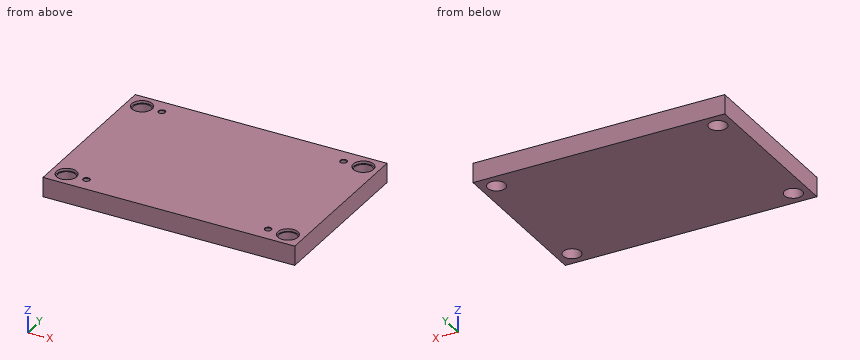
from build123d import *

# Parameters (mm, degrees)
SZKIC1_W                    = 596
SZKIC1_H                    = 396
DODANIE_WYCI_GNI_CIE1_DEPTH = 46
SZKIC2_R                    = 21
WYTNIJ_WYCI_GNI_CIE1_DEPTH  = 46
SZKIC3_R                    = 21
WYTNIJ_WYCI_GNI_CIE2_DEPTH  = 46
SZKIC4_R                    = 21
WYTNIJ_WYCI_GNI_CIE3_DEPTH  = 46
SZKIC5_R                    = 21
WYTNIJ_WYCI_GNI_CIE4_DEPTH  = 46
SZKIC6_R                    = 24
WYTNIJ_WYCI_GNI_CIE5_DEPTH  = 6.3
SZKIC7_R                    = 24
WYTNIJ_WYCI_GNI_CIE6_DEPTH  = 6.3
SZKIC8_R                    = 24
WYTNIJ_WYCI_GNI_CIE7_DEPTH  = 6.3
SZKIC9_R                    = 24
WYTNIJ_WYCI_GNI_CIE8_DEPTH  = 6.3


with BuildPart() as part:
    # Szkic1 → Dodanie-wyci_gni_cie1 (new body)
    with BuildSketch(Plane.XY):
        Rectangle(SZKIC1_W, SZKIC1_H)
    extrude(amount=DODANIE_WYCI_GNI_CIE1_DEPTH)

    # Szkic2 → Wytnij-wyci_gni_cie1 (cut)
    with BuildSketch(Plane.XY.offset(46)):
        with Locations((262, 162)):
            Circle(SZKIC2_R)
    extrude(amount=-WYTNIJ_WYCI_GNI_CIE1_DEPTH, mode=Mode.SUBTRACT)

    # Szkic3 → Wytnij-wyci_gni_cie2 (cut)
    with BuildSketch(Plane.XY.offset(46)):
        with Locations((262, -162)):
            Circle(SZKIC3_R)
    extrude(amount=-WYTNIJ_WYCI_GNI_CIE2_DEPTH, mode=Mode.SUBTRACT)

    # Szkic4 → Wytnij-wyci_gni_cie3 (cut)
    with BuildSketch(Plane.XY.offset(46)):
        with Locations((-262, -162)):
            Circle(SZKIC4_R)
    extrude(amount=-WYTNIJ_WYCI_GNI_CIE3_DEPTH, mode=Mode.SUBTRACT)

    # Szkic5 → Wytnij-wyci_gni_cie4 (cut)
    with BuildSketch(Plane.XY.offset(46)):
        with Locations((-262, 162)):
            Circle(SZKIC5_R)
    extrude(amount=-WYTNIJ_WYCI_GNI_CIE4_DEPTH, mode=Mode.SUBTRACT)

    # Szkic6 → Wytnij-wyci_gni_cie5 (cut)
    with BuildSketch(Plane.XY.offset(46)):
        with Locations((-262, 162)):
            Circle(SZKIC6_R)
    extrude(amount=-WYTNIJ_WYCI_GNI_CIE5_DEPTH, mode=Mode.SUBTRACT)

    # Szkic7 → Wytnij-wyci_gni_cie6 (cut)
    with BuildSketch(Plane.XY.offset(46)):
        with Locations((262, 162)):
            Circle(SZKIC7_R)
    extrude(amount=-WYTNIJ_WYCI_GNI_CIE6_DEPTH, mode=Mode.SUBTRACT)

    # Szkic8 → Wytnij-wyci_gni_cie7 (cut)
    with BuildSketch(Plane.XY.offset(46)):
        with Locations((-262, -162)):
            Circle(SZKIC8_R)
    extrude(amount=-WYTNIJ_WYCI_GNI_CIE7_DEPTH, mode=Mode.SUBTRACT)

    # Szkic9 → Wytnij-wyci_gni_cie8 (cut)
    with BuildSketch(Plane.XY.offset(46)):
        with Locations((262, -162)):
            Circle(SZKIC9_R)
    extrude(amount=-WYTNIJ_WYCI_GNI_CIE8_DEPTH, mode=Mode.SUBTRACT)

    # Szkic10 → Wyci_cie-obr_t1 (revolve, cut)
    with BuildSketch(Plane(origin=(-215, 0, 0), x_dir=(0, 0, -1), z_dir=(1, 0, 0)), mode=Mode.PRIVATE) as wyci_cie_obr_t1_sk:
        Polygon((-46, 162), (-46, 170), (-44.9175, 168.9175), (-6, 168.9175), (-2.006179513, 162), align=None)
    revolve(wyci_cie_obr_t1_sk.sketch.rotate(Axis((-215, 162, 2.006179513), (0, 0, 1)), 270), axis=Axis((-215, 162, 2.006179513), (0, 0, 1)), mode=Mode.SUBTRACT)

    # Szkic11 → Wyci_cie-obr_t2 (revolve, cut)
    with BuildSketch(Plane(origin=(-215, 0, 0), x_dir=(0, 0, -1), z_dir=(1, 0, 0)), mode=Mode.PRIVATE) as wyci_cie_obr_t2_sk:
        Polygon((-2.006179513, -162), (-6, -168.9175), (-44.9175, -168.9175), (-46, -170), (-46, -162), align=None)
    revolve(wyci_cie_obr_t2_sk.sketch.rotate(Axis((-215, -162, 46), (0, 0, -1)), 90), axis=Axis((-215, -162, 46), (0, 0, -1)), mode=Mode.SUBTRACT)

    # Szkic12 → Wyci_cie-obr_t3 (revolve, cut)
    with BuildSketch(Plane(origin=(215, 0, 0), x_dir=(0, 0, -1), z_dir=(1, 0, 0)), mode=Mode.PRIVATE) as wyci_cie_obr_t3_sk:
        Polygon((-46, 162), (-46, 170), (-44.9175, 168.9175), (-6, 168.9175), (-2.006179513, 162), align=None)
    revolve(wyci_cie_obr_t3_sk.sketch.rotate(Axis((215, 162, 2.006179513), (0, 0, 1)), 270), axis=Axis((215, 162, 2.006179513), (0, 0, 1)), mode=Mode.SUBTRACT)

    # Szkic13 → Wyci_cie-obr_t4 (revolve, cut)
    with BuildSketch(Plane(origin=(215, 0, 0), x_dir=(0, 0, -1), z_dir=(1, 0, 0)), mode=Mode.PRIVATE) as wyci_cie_obr_t4_sk:
        Polygon((-2.006179513, -162), (-6, -168.9175), (-44.9175, -168.9175), (-46, -170), (-46, -162), align=None)
    revolve(wyci_cie_obr_t4_sk.sketch.rotate(Axis((215, -162, 46), (0, 0, -1)), 90), axis=Axis((215, -162, 46), (0, 0, -1)), mode=Mode.SUBTRACT)


solid = part.part
Geometry: final body of the model. Coordinates: model frame, mm. Coordinates: 2 decimals unless noted, no trailing zeros. Write each loop counter-clockwise with the first axis right and the second up, starting at its lowest first coordinate (ties: lowest second). Pieces come first, ordered by that corner, then holes. Notation, with made-up numbers: (-17.75, 51.5) - (-1.75, 51.5) arc R25 ccw to (-1.75, 82.5) - close; hole circle Ø10 at (61.25, 37). An arc over 180 degrees is marked (long way). Return JSON: item names as keys, results as strings.
Item 1: Section query B-B (x = 262). Output: boundary loops of the cut face in (y, z), and give its area (3 significant figures).
Completed:
{"outline": "(-198, 0) - (-183, 0) - (-183, 39.7) - (-186, 39.7) - (-186, 46) - (-198, 46) - close; (-141, 0) - (141, 0) - (141, 39.7) - (138, 39.7) - (138, 46) - (-138, 46) - (-138, 39.7) - (-141, 39.7) - close; (183, 0) - (198, 0) - (198, 46) - (186, 46) - (186, 39.7) - (183, 39.7) - close", "area": "14,300 mm2"}
Item 2: Line query: L1, parallel to Y at x = 215, z = 26; L2, parallel to Y at x = 262, z = 42; L3, parallel to X at y = 159, z = 25. Output: solid intervals per line, ascending.
Completed:
{"L1": "y = -198 to -168.92, -155.08 to 155.08, 168.92 to 198", "L2": "y = -198 to -186, -138 to 138, 186 to 198", "L3": "x = -298 to -282.78, -241.22 to -221.23, -208.77 to 208.77, 221.23 to 241.22, 282.78 to 298"}
Item 3: Section query A-A (z = 15). Count the separate pieces of the cut face and the enclosed holes in it, and give its area (3 significant figures).
Completed:
{"separate pieces": "1", "enclosed holes": "8", "area": "230,000 mm2"}
